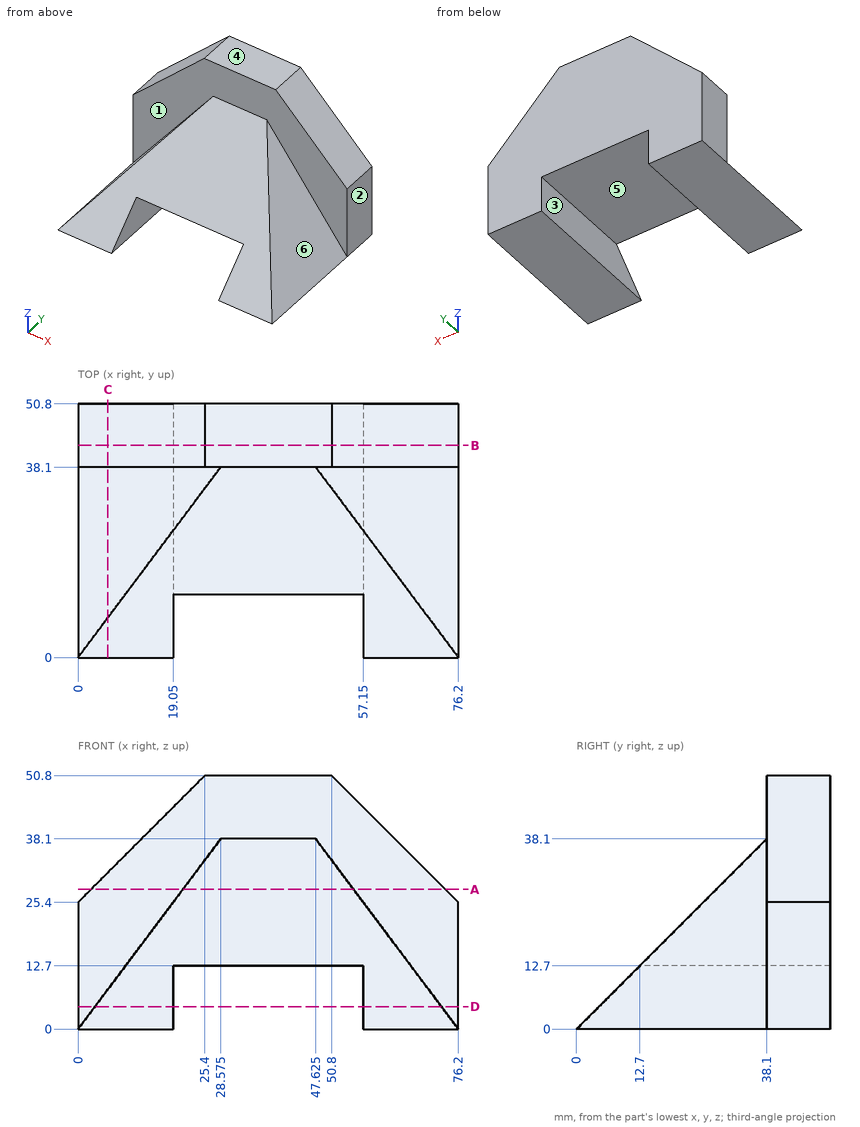
Here's the drawing with two shaded views (mm, measured from the low corner). I have some questions. A direction names the side the tool comes from. Give positions to 0.01 mm unless a question says otherwise; leave off trailing zeros. Order: outer loops, then holes, each group sorted by start corner. A loop starts at its lowest first (then second) coordinate and runs counter-clockwise, first axis right, second up. Notation, with made-up numbers: (71.5, 87) -> (88.5, 87) arc R22 cw to (88.5, 108) -> close; hole circle Ø6 at (6, 39). An arc over 180 degrees is marked (long way). Use a Markdown table: item, result. Add a question column.
Item 1: Will these pins go through, and if not, where does the flat tip stop? pin 1 (12 mm diameter, centred on x = 30.5, z = 29, fed in from -Y); pin 2 (1.5 mm diameter, centred on x = 53, z = 14.5, fed in from -Y); pin 3 (12 mm diameter, centred on y = 40.5, z = 34, fed in from -X).
Item 2: Imagine slicing it at A-A on z = 28. Please give me the cut outline in (x, y), plus the area to 3 significant figures.
Item 3: Imagine slicing it at D-D on z = 4.5. Please give me the cut outline in (x, y) (3 decimals).
Item 4: For the marked faces 1, 2 and 3, which set-ups out of +Z, -Z, +X, -X, +Y, -Y let a thin tool reach every point of the face, with its end or its side?
Item 5: If we mould it in two halves opening along X, with no side actions, what happens to the marked faces 4, 5 and 6? For each: pulls with the +X half, pulls with the -X half, needs draft (parallel to the pull), parting line crosses it, or undercut.
Item 6: Imagine slicing it at C-C on x = 6. Please give me the cut outline in (y, z).
Item 7: Imagine slicing it at B-B on y = 42.5. Please give me the cut outline in (x, z).
Item 8: I need wall thicknesses on line 1 (X direction, y = 23.5, z = 4); line 2 (Y direction, x = 17.5, z = 27.5); line 3 (X direction, y = 34.5, z = 8). Which ranges of each line are inside material? Lowest first, please.
Data:
| question | item | result |
|---|---|---|
| 1 | pin 1 | stops at y = 23 |
| 1 | pin 2 | stops at y = 13.75 |
| 1 | pin 3 | stops at x = 2.6 |
| 2 | outline | (2.6, 38.1) -> (21, 38.1) -> (21, 28) -> (55.2, 28) -> (55.2, 38.1) -> (73.6, 38.1) -> (73.6, 50.8) -> (2.6, 50.8) -> close |
| 2 | area | 1,250 mm² |
| 3 | outline | (0, 38.1) -> (3.375, 38.1) -> (3.375, 4.5) -> (19.05, 4.5) -> (19.05, 50.8) -> (0, 50.8) -> close; (57.15, 4.5) -> (72.825, 4.5) -> (72.825, 38.1) -> (76.2, 38.1) -> (76.2, 50.8) -> (57.15, 50.8) -> close |
| 4 | face 1 | +Z, -Y |
| 4 | face 2 | +Z, -Z, +X, +Y, -Y |
| 4 | face 3 | -Z, +Y, -Y |
| 5 | face 4 | needs draft |
| 5 | face 5 | undercut |
| 5 | face 6 | pulls with the +X half |
| 6 | outline | (0, 0) -> (50.8, 0) -> (50.8, 31.4) -> (38.1, 31.4) -> (38.1, 8) -> (8, 8) -> close |
| 7 | outline | (0, 0) -> (19.05, 0) -> (19.05, 12.7) -> (57.15, 12.7) -> (57.15, 0) -> (76.2, 0) -> (76.2, 25.4) -> (50.8, 50.8) -> (25.4, 50.8) -> (0, 25.4) -> close |
| 8 | line 1 | x = 3 to 19.05, 57.15 to 73.2 |
| 8 | line 2 | y = 38.1 to 50.8 |
| 8 | line 3 | x = 6 to 19.05, 57.15 to 70.2 |
